Source: CAD feature listing. Evaluate the final solid. Frame: model axes, mm. A direction names the side the tool comes from. Give positions to 0.01 mm unless a question says otherwise; leave off trailing zeros. Loops run counter-clockwise (first coordinate to the right, second up) from the corner with the lowest first, then second, coordinate; pieces in that order, holes last. Notation, with made-up numbers: (-31.5, 11.25) - (25.5, 11.25) arc R13 cw to (25.5, 16.25) - close; hole circle Ø3 at (27, 55). An arc over 180 degrees is marked (long way). Put each result on its own line as item: value.
```python
from build123d import *

# Parameters (mm, degrees)
SKETCH1_R                = 2.75
BOSS_EXTRUDE1_DEPTH      = 5
BOSS_EXTRUDE2_DEPTH      = 25
BOSS_EXTRUDE2_DEPTH_BACK = 5
SKETCH2_W                = 60
SKETCH2_H                = 6
SKETCH3_W                = 60
SKETCH3_H                = 10
BOSS_EXTRUDE3_DEPTH      = 167.8942
SKETCH4_W                = 60
SKETCH4_H                = 5
BOSS_EXTRUDE4_DEPTH      = 50
SKETCH5_W                = 60
SKETCH5_H                = 10
BOSS_EXTRUDE5_DEPTH      = 25.4
M5X0_8_TAPPED_HOLE1_D    = 5


with BuildPart() as part:
    # Sketch1 → Boss-Extrude1 (new body)
    # profile 1 of 2: a face of its own
    with BuildSketch(Plane.XY):
        Polygon((13, 7.5), (13, 32.5), (0, 32.5), (0, 0), (30, 0), (30, 7.5), align=None)
        with Locations((7, 7)):
            Circle(SKETCH1_R, mode=Mode.SUBTRACT)
        with Locations((7, 25)):
            Circle(SKETCH1_R, mode=Mode.SUBTRACT)
    # profile 2 of 2: a face of its own
    with BuildSketch(Plane.XY):
        Polygon((47, 7.5), (30, 7.5), (30, 0), (60, 0), (60, 32.5), (47, 32.5), align=None)
        with Locations((53, 7)):
            Circle(SKETCH1_R, mode=Mode.SUBTRACT)
        with Locations((53, 25)):
            Circle(SKETCH1_R, mode=Mode.SUBTRACT)
    extrude(amount=BOSS_EXTRUDE1_DEPTH)

    # Sketch2 → Boss-Extrude2 (add, two sides: drawn at the far end of the back side and taken through both)
    with BuildSketch(Plane.XY.offset(5).offset(-BOSS_EXTRUDE2_DEPTH_BACK)):
        with Locations((30, -3)):
            Rectangle(SKETCH2_W, SKETCH2_H)
    extrude(amount=BOSS_EXTRUDE2_DEPTH + BOSS_EXTRUDE2_DEPTH_BACK)

    # Sketch3 → Boss-Extrude3 (add)
    with BuildSketch(Plane(origin=(0, 0, 0), x_dir=(-1, 0, 0), z_dir=(0, 0, -1))):
        with Locations((-30, -11)):
            Rectangle(SKETCH3_W, SKETCH3_H)
    extrude(amount=-BOSS_EXTRUDE3_DEPTH)

    # Sketch4 → Boss-Extrude4 (add)
    with BuildSketch(Plane(origin=(0, -6, 0), x_dir=(1, 0, 0), z_dir=(0, 1, 0))):
        with Locations((30, -165.3942)):
            Rectangle(SKETCH4_W, SKETCH4_H)
    extrude(amount=BOSS_EXTRUDE4_DEPTH)

    # Sketch5 → Boss-Extrude5 (add)
    with BuildSketch(Plane.XY.offset(167.8942)):
        with Locations((30, 33.0996)):
            Rectangle(SKETCH5_W, SKETCH5_H)
    extrude(amount=BOSS_EXTRUDE5_DEPTH)

    # M5x0.8 Tapped Hole1 (through all)
    with Locations(Plane(origin=(0, 38.0996, 0), x_dir=(1, 0, 0), z_dir=(0, 1, 0))):
        with Locations((45, -180.5942), (15, -180.5942)):
            Hole(M5X0_8_TAPPED_HOLE1_D / 2)


solid = part.part
```
1) Section query A-A, the plane y = -2.5. Output: boundary loops of the cut face in (x, z), plus the area to 3 significant figures.
Check result:
outline: (0, 0) - (60, 0) - (60, 30) - (0, 30) - close; (0, 162.89) - (60, 162.89) - (60, 167.89) - (0, 167.89) - close
area: 2,100 mm²
2) Mould query, pull axis Z, two halves, no side actions, for faces 6 (the flat face through (30, 38.1, 180)), 7 (the flat face through (30, 19, 162.894)), 8 (the flat face through (30, 33, 193.294)). Classes: pulls with the +Z half, pulls with the -Z half, needs draft (parallel to the pull), parting line crosses it, or undercut.
Check result:
face 6: needs draft
face 7: undercut
face 8: pulls with the +Z half
3) Section query B-B, the plane x = 15. Output: boundary loops of the cut face in (y, z), plus the area to 3 significant figures.
Check result:
outline: (-16, 0) - (7.5, 0) - (7.5, 5) - (0, 5) - (0, 30) - (-6, 30) - (-6, 162.89) - (44, 162.89) - (44, 167.89) - (38.1, 167.89) - (38.1, 178.09) - (28.1, 178.09) - (28.1, 167.89) - (-16, 167.89) - close; (28.1, 183.09) - (38.1, 183.09) - (38.1, 193.29) - (28.1, 193.29) - close
area: 2,350 mm²
4) Material intervals for line 1 along Y through (x, z) = (7, 2.65); line 2 along Z through (x, y) = (45, 32); line 3 along Z through (x, y) = (23.5, 4.5), sorted ascending. Write a range as [from, to].
Check result:
line 1: [-16, 4.25], [9.75, 22.25], [27.75, 32.5]
line 2: [162.89, 178.09], [183.09, 193.29]
line 3: [0, 5], [162.89, 167.89]
5) Section query D-D, the plane x = 31. Output: boundary loops of the cut face in (y, z), plus the area to 3 significant figures.
Check result:
outline: (-16, 0) - (7.5, 0) - (7.5, 5) - (0, 5) - (0, 30) - (-6, 30) - (-6, 162.89) - (44, 162.89) - (44, 167.89) - (38.1, 167.89) - (38.1, 193.29) - (28.1, 193.29) - (28.1, 167.89) - (-16, 167.89) - close
area: 2,400 mm²
6) Pin query (flat end, axial travel): P1, Ø1.8, axis at x = 39.5, y = 41.5, coming from the +Z side; P2, Ø8, axis at x = 15, z = 180.59, coming from the +Y side; P3, Ø2.5, axis at x = 52, z = 3, coming from the +Y side; P4, Ø5.5, axis at y = 16, z = 2.5, coming from the -X side. Return the tip coordinate at first contact, or that it passes through.
Check result:
P1: z = 167.89
P2: y = 38.1
P3: y = 32.5
P4: x = 0
7) Section query C-C, the plane x = 7. Output: boundary loops of the cut face in (y, z).
Check result:
outline: (-16, 0) - (4.25, 0) - (4.25, 5) - (0, 5) - (0, 30) - (-6, 30) - (-6, 162.89) - (44, 162.89) - (44, 167.89) - (38.1, 167.89) - (38.1, 193.29) - (28.1, 193.29) - (28.1, 167.89) - (-16, 167.89) - close; (9.75, 0) - (22.25, 0) - (22.25, 5) - (9.75, 5) - close; (27.75, 0) - (32.5, 0) - (32.5, 5) - (27.75, 5) - close
8) Access query for faces 1 (the flat face through (7, 32.5, 2)), 2 (the cylindrical face through (6.642, 27.727, 2.465)), 3 (the flat face through (30, -3, 30)), 4 (the flat face through (13, 20, 2)), 5 (the flat face through (30, 28.1, 180)). Directions: +Z, -Z, +X, -X, +Y, -Y. A direction counts if a zero-diameter tool reaches every point of the face in a straight line with its end or side. Return the directions, or none.
Check result:
face 1: -Z, +X, -X, +Y
face 2: -Z
face 3: +X, -X, +Y
face 4: -Z, +Y
face 5: +Z, +X, -X, -Y
